For this review, take the finished solid that the model builds, in its own axes (mm). A direction names the side the tool comes from. Coordinates: 2 decimals unless noted, no trailing zeros. Loops run counter-clockwise (first coordinate to the right, second up) from the corner with the lowest first, then second, coordinate; pieces in that order, holes last. Notation, with made-up numbers: (-10, -12) - (7, -12) arc R20 ccw to (7, 27) - close; hole circle Ø7 at (-27, 10.25). An arc over 180 degrees is marked (long way). Answer as a JSON object with one key per item and string values. Group by question number.
Item 1: We need section C-C (y = 25.4). Give the boundary of the cut face in (x, z).
Item 2: Mouldability with a two-part tool opening along Z and no side actions: class faces 1 (the cylindrical face through (-11.172, 75.133, 11.251)), 2 (the flat face through (-11.43, 75, 0)), 3 (the cylindrical face through (-0.47, 28.99, -12.06)), 4 (the cylindrical face through (-12.07, 64.79, -0.78)) as released by +Z, released by -Z, zero draft, split by the parting line, or undercut.
Item 3: Clearance check with flat-ended pins moving along their axes: pin 1 (10 mm diameter, centred on x = 0.5, y = 90.5, fed in from -Z); pin 2 (6 mm diameter, centred on x = 0, y = 88.9, fed in from -Z). State where each tip first meets the part, or that it passes through.
Item 4: Tool access review of faces 5 (the flat face through (0, 75, 11.43)), 6 (the flat face through (-12.7, 75, 0)): name each direction out of +Z, -Z, +X, -X, +Y, -Y from which nothing blocks a thin tool from reaching the whole face with its end or side.
Item 5: We need section A-A (x = 0). Give the boundary of the cut face in (y, z), then the cut area to 3 significant figures.
Item 6: To check wall thickness, follow line 1 (Y direction, x = -12.4, z = 0); line 2 (Y direction, x = 0, z = 12); line 3 (X direction, y = 88.5, z = 3). State the ranges of each line that lie inside material, in increasing order.
Item 7: We need section D-D (y = 62). Give the boundary of the cut face in (x, z), then the cut area to 3 significant figures.
Item 8: We need section B-B (z = 6.25). Give the boundary of the cut face in (x, y), then the cut area to 3 significant figures.
from build123d import *

# Parameters (mm, degrees)
BOSS_EXTRUDE1_DEPTH = 152.4
SKETCH2_R           = 3.6195
CUT_EXTRUDE1_DEPTH  = 26.4
SKETCH3_R           = 3.6195
CUT_EXTRUDE2_DEPTH  = 26.4


with BuildPart() as part:
    # Sketch1 → Boss-Extrude1 (new body)
    with BuildSketch(Plane(origin=(0, 0, 0), x_dir=(1, 0, 0), z_dir=(0, 1, 0))):
        with BuildLine():
            Line((-7.62, 12.7), (7.62, 12.7))
            ThreePointArc((7.62, 12.7), (11.212102448, 11.212102448), (12.7, 7.62))
            Line((12.7, 7.62), (12.7, -7.62))
            ThreePointArc((12.7, -7.62), (11.212102448, -11.212102448), (7.62, -12.7))
            Line((7.62, -12.7), (-7.62, -12.7))
            ThreePointArc((-7.62, -12.7), (-11.212102448, -11.212102448), (-12.7, -7.62))
            Line((-12.7, -7.62), (-12.7, 7.62))
            ThreePointArc((-12.7, 7.62), (-11.212102448, 11.212102448), (-7.62, 12.7))
        make_face()
        with BuildLine():
            Line((-7.62, 11.43), (7.62, 11.43))
            ThreePointArc((7.62, 11.43), (10.314076836, 10.314076836), (11.43, 7.62))
            Line((11.43, 7.62), (11.43, -7.62))
            ThreePointArc((11.43, -7.62), (10.314076836, -10.314076836), (7.62, -11.43))
            Line((7.62, -11.43), (-7.62, -11.43))
            ThreePointArc((-7.62, -11.43), (-10.314076836, -10.314076836), (-11.43, -7.62))
            Line((-11.43, -7.62), (-11.43, 7.62))
            ThreePointArc((-11.43, 7.62), (-10.314076836, 10.314076836), (-7.62, 11.43))
        make_face(mode=Mode.SUBTRACT)
    extrude(amount=BOSS_EXTRUDE1_DEPTH)

    # Sketch2 → Cut-Extrude1 (cut, through all)
    with BuildSketch(Plane.XY.offset(12.7)):
        with Locations((0, 88.9)):
            Circle(SKETCH2_R)
        with Locations((0, 25.4)):
            Circle(SKETCH2_R)
    extrude(amount=-CUT_EXTRUDE1_DEPTH, mode=Mode.SUBTRACT)

    # Sketch3 → Cut-Extrude2 (cut, through all)
    with BuildSketch(Plane.ZY.offset(12.7)):
        with Locations((0, 68.326)):
            Circle(SKETCH3_R)
        with Locations((0, 17.526)):
            Circle(SKETCH3_R)
    extrude(amount=-CUT_EXTRUDE2_DEPTH, mode=Mode.SUBTRACT)


solid = part.part
Check sheet entries:
{
 "1": {"outline": "(-12.7, -7.62) arc R5.08 ccw to (-7.62, -12.7) - (-3.62, -12.7) - (-3.62, -11.43) - (-7.62, -11.43) arc R3.81 cw to (-11.43, -7.62) - (-11.43, 7.62) arc R3.81 cw to (-7.62, 11.43) - (-3.62, 11.43) - (-3.62, 12.7) - (-7.62, 12.7) arc R5.08 ccw to (-12.7, 7.62) - close; (3.62, -12.7) - (7.62, -12.7) arc R5.08 ccw to (12.7, -7.62) - (12.7, 7.62) arc R5.08 ccw to (7.62, 12.7) - (3.62, 12.7) - (3.62, 11.43) - (7.62, 11.43) arc R3.81 cw to (11.43, 7.62) - (11.43, -7.62) arc R3.81 cw to (7.62, -11.43) - (3.62, -11.43) - close"},
 "2": {"face 1": "released by +Z", "face 2": "undercut", "face 3": "zero draft", "face 4": "undercut"},
 "3": {"pin 1": "stops at z = -12.7", "pin 2": "passes through"},
 "4": {"face 5": "+Y, -Y", "face 6": "+Z, -Z, -X, +Y, -Y"},
 "5": {"outline": "(0, -12.7) - (21.78, -12.7) - (21.78, -11.43) - (0, -11.43) - close; (0, 11.43) - (21.78, 11.43) - (21.78, 12.7) - (0, 12.7) - close; (29.02, -12.7) - (85.28, -12.7) - (85.28, -11.43) - (29.02, -11.43) - close; (29.02, 11.43) - (85.28, 11.43) - (85.28, 12.7) - (29.02, 12.7) - close; (92.52, -12.7) - (152.4, -12.7) - (152.4, -11.43) - (92.52, -11.43) - close; (92.52, 11.43) - (152.4, 11.43) - (152.4, 12.7) - (92.52, 12.7) - close", "area": "350 mm2"},
 "6": {"line 1": "y = 0 to 13.91, 21.15 to 64.71, 71.95 to 152.4", "line 2": "y = 0 to 21.78, 29.02 to 85.28, 92.52 to 152.4", "line 3": "x = -12.7 to -11.43, 11.43 to 12.7"},
 "7": {"outline": "(-12.7, -7.62) arc R5.08 ccw to (-7.62, -12.7) - (7.62, -12.7) arc R5.08 ccw to (12.7, -7.62) - (12.7, 7.62) arc R5.08 ccw to (7.62, 12.7) - (-7.62, 12.7) arc R5.08 ccw to (-12.7, 7.62) - close; hole (-11.43, -7.62) arc R3.81 ccw to (-7.62, -11.43) - (7.62, -11.43) arc R3.81 ccw to (11.43, -7.62) - (11.43, 7.62) arc R3.81 ccw to (7.62, 11.43) - (-7.62, 11.43) arc R3.81 ccw to (-11.43, 7.62) - close", "area": "113 mm2"},
 "8": {"outline": "(-12.7, 0) - (-11.43, 0) - (-11.43, 152.4) - (-12.7, 152.4) - close; (11.43, 0) - (12.7, 0) - (12.7, 152.4) - (11.43, 152.4) - close", "area": "387 mm2"}
}
